The model under review builds one solid part; all positions refer to its coordinate system, in mm. Face numbers are marked on the shaded views. A direction names the side the tool comes from. Give positions to 0.01 mm unless a question says otherwise; leave off trailing zeros. Loops run counter-clockwise (first coordinate to the right, second up) from the corner with the lowest first, then second, coordinate; pieces in that order, holes last. Notation, with made-up numbers: (-18.5, -30) -> (13.5, -30) arc R35 cw to (13.5, 5) -> close; hole circle Ø7 at (5.25, -26.75). An arc over 180 degrees is marked (long way). Write each question's results on one line, items separated by ' | '. Start each with the question number.
Q1. We need section B-B (x = -16.5). Write out the cut boundary in (y, z).
Q2. Wall thickness on L1, parallel to Y at x = 63, z = -1; L2, parallel to X at y = 9, z = 16.5; L3, parallel to X at y = -2.5, z = 15.5: over which ranges is each line inside the solid? List them lowest first. Write a range as [from, to].
Q3. Insertion check: pin 1 Ø1.7 at (x, z) = (10.5, 16.5) entering from -Y; pin 2 Ø1 at (x, z) = (40.5, -5.5) entering from -Y; pin 3 Ø8 at (x, y) = (-30, -3.5) entering from -Z. Each pin has a flat end and moves straight along its axis. Give the tip position at first contact, or say it passes through.
Q4. We need section A-A (z = 0). Write out the cut boundary in (x, y), plus the area to 3 significant figures.
Q5. We need section C-C (x = -68). Write out the cut boundary in (y, z).
Q6. Machinability: for the marked faces 1, 2 and 3, which of the approach directions +Z, -Z, +X, -X, +Y, -Y give a long, thin tool a straight path to every point of the face, cutting with its end or side? Answer none if there is none.
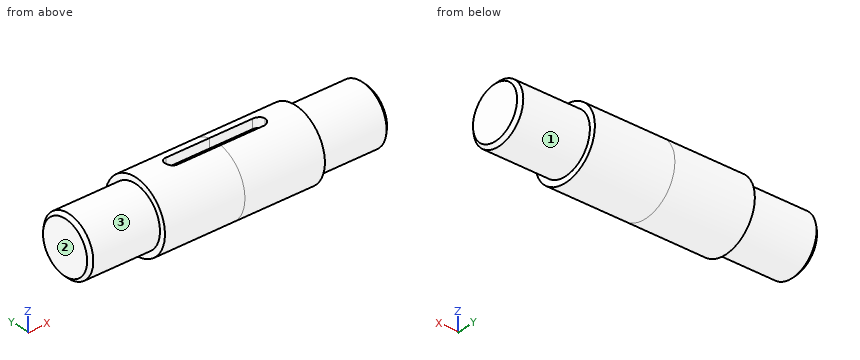
from build123d import *

# Parameters (mm, degrees)
F0_R     = 21
F1_DEPTH = 48
F2_R     = 17.5
F3_DEPTH = 42
F4_SIZE  = 2
F5_W     = 8
F5_H     = 12
F6_DEPTH = 30
F7_R     = 3.999


# Not quite as in the source:
# - a fillet or chamfer is up to 0.001 mm smaller than in the source, because OpenCascade refuses the exact size


with BuildPart() as f1:
    # F0 (on Right) → F1 (new body)
    with BuildSketch(Plane.YZ):
        Circle(F0_R)
    extrude(amount=F1_DEPTH)

    # F2 (on face) → F3 (join)
    with BuildSketch(Plane.YZ.offset(48)):
        Circle(F2_R)
    extrude(amount=F3_DEPTH)

    # F4
    f4_edges = [f1.edges().sort_by_distance(p)[0] for p in [
        (90, -17.5, 0),
    ]]
    chamfer(f4_edges, length=F4_SIZE)

    # F5 (on face) → F6 (cut)
    with BuildSketch(Plane(origin=(0, 0, 0), x_dir=(0, -1, 0), z_dir=(-1, 0, 0))):
        with Locations((0, 21)):
            Rectangle(F5_W, F5_H)
    extrude(amount=-F6_DEPTH, mode=Mode.SUBTRACT)

    # F7 (radius 4 in the source; OpenCascade refuses exactly that, so slightly less here)
    f7_edges = [f1.edges().sort_by_distance(p)[0] for p in [
        (30, 4, 17.807764),
        (30, -4, 17.807764),
    ]]
    fillet(f7_edges, radius=F7_R)

    # F8: F1 across face


with BuildPart() as f1_1:
    add(f1.part)
    add(f1.part.mirror(Plane(origin=(0, 0, -0.629577464), x_dir=(0, 1, 0), z_dir=(-1, 0, 0))))


solid = f1_1.part
Output:
1) outline: (-4, 15) -> (-4, 20.62) arc R21 ccw (long way) to (4, 20.62) -> (4, 15) -> close
2) L1: [-17.47, 17.47] | L2: [-48, 48] | L3: [-89.8, -29.12], [29.12, 89.8]
3) pin 1: y = -14 | pin 2: y = -20.4 | pin 3: z = -21
4) outline: (-90, -15.5) -> (-88, -17.5) -> (-48, -17.5) -> (-48, -21) -> (48, -21) -> (48, -17.5) -> (88, -17.5) -> (90, -15.5) -> (90, 15.5) -> (88, 17.5) -> (48, 17.5) -> (48, 21) -> (-48, 21) -> (-48, 17.5) -> (-88, 17.5) -> (-90, 15.5) -> close | area: 6,960 mm2
5) outline: circle Ø35 at (0, 0)
6) face 1: +X | face 2: +Z, -Z, -X, +Y, -Y | face 3: -X
